Verification items for the finished model (mm, model axes). A direction names the side the tool comes from. Give positions to 0.01 mm unless a question says otherwise; leave off trailing zeros. Write each loop counter-clockwise with the first axis right and the second up, starting at its lowest first coordinate (ties: lowest second). Pieces come first, ordered by that corner, then holes. Notation, with made-up numbers: M 62,30.5 L 89,30.5 A32 cw 89,67.5 Z; hole C 26,2.25 d9. An arc over 180 degrees is marked long. Write item = value, one per line.
Autodesk Inventor part; units mm, degrees
ref_plane "YZ Plane" through (0, 0, 0) normal (1, 0, 0) x (0, 1, 0)
ref_plane "XZ Plane" through (0, 0, 0) normal (0, 1, 0) x (-1, 0, 0)
ref_plane "XY Plane" through (0, 0, 0) normal (0, 0, 1) x (1, 0, 0)
sketch "Bracket Short" plane through (0, 0, 0) normal (0, 0, 1) x (1, 0, 0)
  line L0 (0, 0) -> (30, 0)
  line L1 (25, 10) -> (0, 10)
  line L2 (0, 10) -> (0, 0)
  line L3 (30, 0) -> (55, 0)
  line L4 (55, 0) -> (55, 40)
  line L5 (55, 40) -> (35, 40)
  line L6 (35, 40) -> (35, 20)
  arc A0 (25, 10) -> (35, 20) centre (25, 20) ccw
  point P0 (35, 10)
  dimension "d0" = 35
  dimension "d2" = 20
  dimension "d3" = 40
  dimension "d4" = 10
  dimension "d10" = 10
extrude "Extrusion1" add sketch "Bracket Short" along normal blind 20
sketch "Clearance Hole (M6-8)" plane through (0, 10, 0) normal (0, 1, 0) x (1, 0, 0)
  circle A0 centre (12.5, -10) radius 5
  point P0 (0, 0)
  dimension "d7" = 10
extrude "Extrusion2" cut sketch "Clearance Hole (M6-8)" against normal through all
sketch "Sketch3" plane through (0, 0, 0) normal (0, 0, -1) x (-1, 0, 0)
  circle A0 centre (-45, 20) radius 2
  point P0 (0, 0)
  dimension "d15" = 4
hole "Hole1" at (45, 20, 0) direction (0, 0, 1) diameter 3.242 depth 11.8 tip angle 118
move faces "Move1" translate (5, 0, 0) faces at (0, 6.6667, 6.6667)
properties part number "Bracket_Short" material "Aluminum, Anodized Silver"
1) Cross-section at D-D on y = 3.5. Record the boundary of the cut face in (x, z), plus the area to 3 significant figures.
From the geometry:
outline = M 5,0 L 55,0 L 55,20 L 5,20 Z; hole C 12.5,10 d10
area = 921 mm^2
2) Depth check by flat-ended pin: P1, Ø1.5, axis at x = 28, z = 17, coming from the +Y side; P2, Ø12, axis at y = 32.5, z = 16.5, coming from the -X side; P3, Ø4, axis at x = 25, z = 6, coming from the +Y side; P4, Ø3, axis at x = 40, z = 5, coming from the -Y side. Enter the tip coordinate at first touch or a pass-through.
From the geometry:
P1 = 10.73
P2 = 35
P3 = 10.2
P4 = 0
3) Cross-section at C-C on z = 2.5. Record the boundary of the cut face in (x, y).
From the geometry:
outline = M 5,0 L 55,0 L 55,40 L 35,40 L 35,20 A10 cw 25,10 L 5,10 Z; hole C 45,20 d3.24
4) Cross-section at A-A on x = 12.5. Record the boundary of the cut face in (y, z).
From the geometry:
outline = M 0,0 L 10,0 L 10,5 L 0,5 Z; M 0,15 L 10,15 L 10,20 L 0,20 Z
5) Cross-section at B-B on z = 10. Record the boundary of the cut face in (x, y), plus the area to 3 significant figures.
From the geometry:
outline = M 5,0 L 7.5,0 L 7.5,10 L 5,10 Z; M 17.5,0 L 55,0 L 55,40 L 35,40 L 35,20 A10 cw 25,10 L 17.5,10 Z; hole C 45,20 d3.24
area = 1,010 mm^2
6) Tool access check on faces 1 (the cylindrical face through (44.513, 21.546, 5.983)), 2 (the flat face through (45, 40, 10)), 3 (the flat face through (35, 30, 10)). Record the directions out of +Z, -Z, +X, -X, +Y, -Y that give a thin tool (end or side, any length) a straight path to the whole face; none if there is none.
From the geometry:
face_1 = -Z
face_2 = +Z, -Z, +X, -X, +Y
face_3 = +Z, -Z, -X, +Y
7) Material ranges on probe 1 along Z at (x, y) = (12.5, 6); probe 2 along X at (y, z) = (2, 10); probe 3 along X at (y, z) = (20, 3.5), recorded low to high. Write a range as from..to.
From the geometry:
probe_1 = 0..5, 15..20
probe_2 = 5..7.5, 17.5..55
probe_3 = 35..43.38, 46.62..55
8) Draft check along X on faces 4 (the flat face through (35, 16, 0)), 5 (the conical face through (44.725, 19.939, 12.605)), 6 (the flat face through (5, 5, 10)). Enter one of: +X half, -X half, draft (parallel to the pull), parting line (faces both ways), or undercut.
From the geometry:
face_4 = draft
face_5 = undercut
face_6 = -X half
